from build123d import *

# Parameters (mm, degrees)
ESBO_O1_R                  = 1.35
RESSALTO_EXTRUS_O1_DEPTH   = 2
ESBO_O3_W                  = 40.2
ESBO_O3_H                  = 2
RESSALTO_EXTRUS_O2_DEPTH   = 10.08
ESBO_O4_W                  = 3.1
ESBO_O4_H                  = 12.84
RESSALTO_EXTRUS_O3_DEPTH   = 34
CORTE_EXTRUS_O1_DEPTH      = 55.735280213
CORTE_EXTRUS_O1_DEPTH_BACK = 55.735280213
ESBO_O5_R                  = 1.35
ESBO_O7_W                  = 37.1
ESBO_O7_H                  = 3.24
CORTE_EXTRUS_O2_DEPTH      = 2
RESSALTO_EXTRUS_O5_START   = 2
ESBO_O12_R                 = 1.35
RESSALTO_EXTRUS_O5_DEPTH   = 2
ESBO_O18_W                 = 3.1
ESBO_O18_H                 = 3.24
RESSALTO_EXTRUS_O6_DEPTH   = 2
ESBO_O19_W                 = 3.1
ESBO_O19_H                 = 3.24
RESSALTO_EXTRUS_O7_DEPTH   = 2
ESBO_O21_R                 = 1.301764144
ESBO_O21_R_2               = 1.35
RESSALTO_EXTRUS_O8_DEPTH   = 1.1
RESSALTO_EXTRUS_O9_START   = 1.1
ESBO_O22_R                 = 1.35
RESSALTO_EXTRUS_O9_DEPTH   = 1.1
ESBO_O23_W                 = 3.1
ESBO_O23_H                 = 5.6
RESSALTO_EXTRUS_O10_DEPTH  = 5.85
CORTE_EXTRUS_O3_REACH      = 63.173
ESBO_O24_R                 = 1.35
ESBO_O25_W                 = 4.5
ESBO_O25_H                 = 3.1
CORTE_EXTRUS_O6_DEPTH      = 4.48
ESBO_O27_W                 = 3.1
ESBO_O27_H                 = 29
CORTE_EXTRUS_O7_DEPTH      = 4.48
ESBO_O28_W                 = 25
ESBO_O28_H                 = 40.2
CORTE_EXTRUS_O8_DEPTH      = 1.24
ESBO_O29_W                 = 25
ESBO_O29_H                 = 5.6
RESSALTO_EXTRUS_O11_DEPTH  = 34
ESBO_O31_W                 = 3.1
ESBO_O31_H                 = 25
RESSALTO_EXTRUS_O12_DEPTH  = 2.84
ESBO_O32_W                 = 25
ESBO_O32_H                 = 5.6
RESSALTO_EXTRUS_O13_DEPTH  = 34
FILETE1_R                  = 2.84
ESBO_O33_W                 = 5.6
ESBO_O33_H                 = 3.1
CORTE_EXTRUS_O9_DEPTH      = 0.55
ESBO_O35_W                 = 3.1
ESBO_O35_H                 = 5.6
CORTE_EXTRUS_O10_DEPTH     = 5.03
FILETE2_R                  = 2.8
DIVIDIR1_SURFACE_1_BACK    = 61.888
DIVIDIR1_SURFACE_1_DEPTH   = 123.776
DIVIDIR1_SURFACE_2_BACK    = 61.888
DIVIDIR1_SURFACE_2_DEPTH   = 123.776


with BuildPart() as part:
    # Esboço1 → Ressalto-extrusão1 (new body)
    with BuildSketch(Plane.XY):
        Polygon((0, 0), (5.6, 0), (5.6, -5.85), (34.6, -5.85), (34.6, 0), (40.2, 0), (40.2, -11.45), (0, -11.45), align=None)
        with Locations((2.8, -3.35)):
            Circle(ESBO_O1_R, mode=Mode.SUBTRACT)
        with Locations((37.4, -3.35)):
            Circle(ESBO_O1_R, mode=Mode.SUBTRACT)
        with Locations((31.1, -8.65)):
            Circle(ESBO_O1_R, mode=Mode.SUBTRACT)
        with Locations((9.1, -8.65)):
            Circle(ESBO_O1_R, mode=Mode.SUBTRACT)
    extrude(amount=RESSALTO_EXTRUS_O1_DEPTH)

    # Esboço3 → Ressalto-extrusão2 (add)
    with BuildSketch(Plane.XZ.offset(11.45)):
        with Locations((20.1, 1)):
            Rectangle(ESBO_O3_W, ESBO_O3_H)
    extrude(amount=RESSALTO_EXTRUS_O2_DEPTH)

    # Esboço4 → Ressalto-extrusão3 (add)
    with BuildSketch(Plane(origin=(0, 0, 0), x_dir=(-1, 0, 0), z_dir=(0, 0, -1))):
        with Locations((-38.65, -15.11)):
            Rectangle(ESBO_O4_W, ESBO_O4_H)
        with Locations((-1.55, -15.11)):
            Rectangle(ESBO_O4_W, ESBO_O4_H)
    extrude(amount=RESSALTO_EXTRUS_O3_DEPTH)

    # Esboço5 → Corte-extrusão1 (cut, two sides: drawn at the far end of the back side and taken through both)
    with BuildSketch(Plane.ZY.offset(-37.1).offset(-CORTE_EXTRUS_O1_DEPTH_BACK)):
        with Locations((-6, -14.25)):
            Circle(ESBO_O5_R)
        with Locations((-28, -14.25)):
            Circle(ESBO_O5_R)
    extrude(amount=CORTE_EXTRUS_O1_DEPTH + CORTE_EXTRUS_O1_DEPTH_BACK, mode=Mode.SUBTRACT)

    # Esboço7 → Corte-extrusão2 (cut)
    with BuildSketch(Plane(origin=(0, 0, 0), x_dir=(-1, 0, 0), z_dir=(0, 0, -1))):
        with Locations((-18.55, -19.91)):
            Rectangle(ESBO_O7_W, ESBO_O7_H)
    extrude(amount=-CORTE_EXTRUS_O2_DEPTH, mode=Mode.SUBTRACT)

    # Esboço12 → Ressalto-extrusão5 (add)
    with BuildSketch(Plane(origin=(0, 0, -34), x_dir=(-1, 0, 0), z_dir=(0, 0, -1)).offset(RESSALTO_EXTRUS_O5_START)):
        Polygon((-5.6, 0), (0, 0), (0, -18.29), (-40.2, -18.29), (-40.2, 0), (-34.6, 0), (-34.6, -5.85), (-5.6, -5.85), align=None)
        with Locations(Location((-31.1, -8.65, 0), (0, 0, 180))):
            Circle(ESBO_O12_R, mode=Mode.SUBTRACT)
        with Locations(Location((-9.1, -8.65, 0), (0, 0, 180))):
            Circle(ESBO_O12_R, mode=Mode.SUBTRACT)
        with Locations(Location((-2.8, -3.35, 0), (0, 0, 180))):
            Circle(ESBO_O12_R, mode=Mode.SUBTRACT)
        with Locations(Location((-37.4, -3.35, 0), (0, 0, 180))):
            Circle(ESBO_O12_R, mode=Mode.SUBTRACT)
    extrude(amount=-RESSALTO_EXTRUS_O5_DEPTH)

    # Esboço18 → Ressalto-extrusão6 (add)
    with BuildSketch(Plane.XY):
        with Locations((1.55, -19.91)):
            Rectangle(ESBO_O18_W, ESBO_O18_H)
    extrude(amount=RESSALTO_EXTRUS_O6_DEPTH)

    # Esboço19 → Ressalto-extrusão7 (add)
    with BuildSketch(Plane(origin=(0, 0, -34), x_dir=(-1, 0, 0), z_dir=(0, 0, -1))):
        with Locations((-1.55, -19.91)):
            Rectangle(ESBO_O19_W, ESBO_O19_H)
        with Locations((-38.65, -19.91)):
            Rectangle(ESBO_O19_W, ESBO_O19_H)
    extrude(amount=RESSALTO_EXTRUS_O7_DEPTH)

    # Esboço21 → Ressalto-extrusão8 (add)
    with BuildSketch(Plane.XY.offset(2)):
        Polygon((37.1, -21.53), (40.2, -21.53), (40.2, 0), (34.6, 0), (34.6, -5.85), (5.6, -5.85), (5.6, 0), (0, 0), (0, -21.53), (3.1, -21.53), (3.1, -18.29), (37.1, -18.29), align=None)
        with Locations((2.8, -3.35)):
            Circle(ESBO_O21_R, mode=Mode.SUBTRACT)
        with Locations((9.1, -8.65)):
            Circle(ESBO_O21_R_2, mode=Mode.SUBTRACT)
        with Locations((31.1, -8.65)):
            Circle(ESBO_O21_R_2, mode=Mode.SUBTRACT)
        with Locations((37.4, -3.35)):
            Circle(ESBO_O21_R_2, mode=Mode.SUBTRACT)
    extrude(amount=RESSALTO_EXTRUS_O8_DEPTH)

    # Esboço22 → Ressalto-extrusão9 (add)
    with BuildSketch(Plane(origin=(0, 0, -36), x_dir=(-1, 0, 0), z_dir=(0, 0, -1)).offset(RESSALTO_EXTRUS_O9_START)):
        Polygon((-5.6, 0), (0, 0), (0, -21.53), (-3.1, -21.53), (-3.1, -18.29), (-37.1, -18.29), (-37.1, -21.53), (-40.2, -21.53), (-40.2, 0), (-34.6, 0), (-34.6, -5.85), (-5.6, -5.85), align=None)
        with Locations(Location((-37.4, -3.35, 0), (0, 0, 180))):
            Circle(ESBO_O22_R, mode=Mode.SUBTRACT)
        with Locations(Location((-31.1, -8.65, 0), (0, 0, 180))):
            Circle(ESBO_O22_R, mode=Mode.SUBTRACT)
        with Locations(Location((-9.1, -8.65, 0), (0, 0, 180))):
            Circle(ESBO_O22_R, mode=Mode.SUBTRACT)
        with Locations(Location((-2.8, -3.35, 0), (0, 0, 180))):
            Circle(ESBO_O22_R, mode=Mode.SUBTRACT)
    extrude(amount=-RESSALTO_EXTRUS_O9_DEPTH)

    # Esboço23 → Ressalto-extrusão10 (add)
    with BuildSketch(Plane.XZ.offset(21.53)):
        with Locations((1.55, 0.3)):
            Rectangle(ESBO_O23_W, ESBO_O23_H)
        with Locations((1.55, -34.3)):
            Rectangle(ESBO_O23_W, ESBO_O23_H)
        with Locations((38.65, -34.3)):
            Rectangle(ESBO_O23_W, ESBO_O23_H)
        with Locations((38.65, 0.3)):
            Rectangle(ESBO_O23_W, ESBO_O23_H)
    extrude(amount=RESSALTO_EXTRUS_O10_DEPTH)

    # Corte-extrusão3: up to this face of the body (flat: up to its plane)
    corte_extrus_o3_end = Plane(part.part.faces().sort_by_distance((40.2, -15.177512698, -17))[0])
    # Esboço24 → Corte-extrusão3 (cut, up to the picked face)
    with BuildSketch(Plane.ZY, mode=Mode.PRIVATE) as corte_extrus_o3_sk1:
        with Locations(Location((-34.3, -19.55, 0), (0, 0, 270))):
            Circle(ESBO_O24_R)
    corte_extrus_o3_tool1 = split(extrude(corte_extrus_o3_sk1.sketch, amount=-CORTE_EXTRUS_O3_REACH, mode=Mode.PRIVATE), bisect_by=corte_extrus_o3_end, keep=Keep.BOTH, mode=Mode.PRIVATE)
    # Esboço24 → Corte-extrusão3 (cut, up to the picked face)
    with BuildSketch(Plane.ZY, mode=Mode.PRIVATE) as corte_extrus_o3_sk2:
        with Locations(Location((0.3, -19.55, 0), (0, 0, 270))):
            Circle(ESBO_O24_R)
    corte_extrus_o3_tool2 = split(extrude(corte_extrus_o3_sk2.sketch, amount=-CORTE_EXTRUS_O3_REACH, mode=Mode.PRIVATE), bisect_by=corte_extrus_o3_end, keep=Keep.BOTH, mode=Mode.PRIVATE)
    add(corte_extrus_o3_tool1.solids().sort_by(Axis((0, -19.55, -34.3), (1, 0, 0)))[0], mode=Mode.SUBTRACT)
    add(corte_extrus_o3_tool2.solids().sort_by(Axis((0, -19.55, 0.3), (1, 0, 0)))[0], mode=Mode.SUBTRACT)

    # Esboço25 → Corte-extrusão6 (cut)
    with BuildSketch(Plane.XZ.offset(18.29)):
        with Locations((5.35, -35.55)):
            Rectangle(ESBO_O25_W, ESBO_O25_H)
        with Locations((34.85, -35.55)):
            Rectangle(ESBO_O25_W, ESBO_O25_H)
        with Locations((34.85, 1.55)):
            Rectangle(ESBO_O25_W, ESBO_O25_H)
        with Locations((5.35, 1.55)):
            Rectangle(ESBO_O25_W, ESBO_O25_H)
    extrude(amount=-CORTE_EXTRUS_O6_DEPTH, mode=Mode.SUBTRACT)

    # Esboço27 → Corte-extrusão7 (cut)
    with BuildSketch(Plane.XZ.offset(21.53)):
        with Locations((1.55, -17)):
            Rectangle(ESBO_O27_W, ESBO_O27_H)
        with Locations((38.65, -17)):
            Rectangle(ESBO_O27_W, ESBO_O27_H)
    extrude(amount=-CORTE_EXTRUS_O7_DEPTH, mode=Mode.SUBTRACT)

    # Esboço28 → Corte-extrusão8 (cut)
    with BuildSketch(Plane.XZ.offset(18.29)):
        with Locations((20.1, -17)):
            Rectangle(ESBO_O28_W, ESBO_O28_H)
    extrude(amount=-CORTE_EXTRUS_O8_DEPTH, mode=Mode.SUBTRACT)

    # Esboço29 → Ressalto-extrusão11 (add)
    with BuildSketch(Plane.XY.offset(-34)):
        with Locations((20.1, -14.25)):
            Rectangle(ESBO_O29_W, ESBO_O29_H)
    extrude(amount=RESSALTO_EXTRUS_O11_DEPTH)

    # Esboço31 → Ressalto-extrusão12 (add)
    with BuildSketch(Plane(origin=(0, -8.69, 0), x_dir=(1, 0, 0), z_dir=(0, 1, 0))):
        with Locations((1.55, 17)):
            Rectangle(ESBO_O31_W, ESBO_O31_H)
        with Locations((38.65, 17)):
            Rectangle(ESBO_O31_W, ESBO_O31_H)
    extrude(amount=RESSALTO_EXTRUS_O12_DEPTH)

    # Esboço32 → Ressalto-extrusão13 (add)
    with BuildSketch(Plane.ZY.offset(-37.1)):
        with Locations((-17, -8.65)):
            Rectangle(ESBO_O32_W, ESBO_O32_H)
    extrude(amount=RESSALTO_EXTRUS_O13_DEPTH)

    # Filete1
    filete1_edges = [part.edges().sort_by_distance(p)[0] for p in [
        (32.6, -17.05, -17),
        (7.6, -17.05, -17),
        (20.1, -5.85, -29.5),
        (20.1, -5.85, -4.5),
    ]]
    fillet(filete1_edges, radius=FILETE1_R)

    # Esboço33 → Corte-extrusão9 (cut)
    with BuildSketch(Plane(origin=(0, 0, 0), x_dir=(1, 0, 0), z_dir=(0, 1, 0))):
        with Locations((2.8, 35.55)):
            Rectangle(ESBO_O33_W, ESBO_O33_H)
        with Locations((37.4, 35.55)):
            Rectangle(ESBO_O33_W, ESBO_O33_H)
        with Locations((37.4, -1.55)):
            Rectangle(ESBO_O33_W, ESBO_O33_H)
        with Locations((2.8, -1.55)):
            Rectangle(ESBO_O33_W, ESBO_O33_H)
    extrude(amount=-CORTE_EXTRUS_O9_DEPTH, mode=Mode.SUBTRACT)

    # Esboço35 → Corte-extrusão10 (cut)
    with BuildSketch(Plane.XZ.offset(27.38)):
        with Locations((1.55, 0.3)):
            Rectangle(ESBO_O35_W, ESBO_O35_H)
        with Locations((38.65, 0.3)):
            Rectangle(ESBO_O35_W, ESBO_O35_H)
        with Locations((38.65, -34.3)):
            Rectangle(ESBO_O35_W, ESBO_O35_H)
        with Locations((1.55, -34.3)):
            Rectangle(ESBO_O35_W, ESBO_O35_H)
    extrude(amount=-CORTE_EXTRUS_O10_DEPTH, mode=Mode.SUBTRACT)

    # Filete2
    filete2_edges = [part.edges().sort_by_distance(p)[0] for p in [
        (34.6, -0.55, 1.55),
        (40.2, -0.55, 1.55),
        (0, -0.55, 1.55),
        (5.6, -0.55, 1.55),
        (40.2, -0.55, -35.55),
        (34.6, -0.55, -35.55),
        (5.6, -0.55, -35.55),
        (0, -0.55, -35.55),
        (1.55, -22.35, -31.5),
        (1.55, -22.35, -37.1),
        (38.65, -22.35, -31.5),
        (38.65, -22.35, -37.1),
        (38.65, -22.35, 3.1),
        (38.65, -22.35, -2.5),
        (1.55, -22.35, -2.5),
        (1.55, -22.35, 3.1),
    ]]
    fillet(filete2_edges, radius=FILETE2_R - 0.0001)  # a hair under: the kernel refuses the full size


with BuildPart() as body_2:
    # Dividir1: the piece behind the surface
    add(part.part)
    # Dividir1 surface: a surface, the sketch's curves swept straight by 123.776 mm
    with BuildLine(Plane.XY.offset(3.1).offset(-DIVIDIR1_SURFACE_1_BACK), mode=Mode.PRIVATE) as dividir1_surface_1_path:
        Line((20.1, -0.55), (20.1, -10.85))
        Line((20.1, -10.85), (17.6, -9.85))
        Line((17.6, -9.85), (17.6, -14.85))
        Line((17.6, -14.85), (20.1, -13.85))
        Line((20.1, -13.85), (20.1, -22.35))
    dividir1_surface_1 = Shell.extrude(dividir1_surface_1_path.wire(), (0 * DIVIDIR1_SURFACE_1_DEPTH, 0 * DIVIDIR1_SURFACE_1_DEPTH, 1 * DIVIDIR1_SURFACE_1_DEPTH))
    split(bisect_by=dividir1_surface_1, keep=Keep.BOTTOM)


with BuildPart() as part_1:
    add(part.part)

    # Dividir1: split by a surface, the side it looks to stays
    # Dividir1 surface: a surface, the sketch's curves swept straight by 123.776 mm
    with BuildLine(Plane.XY.offset(3.1).offset(-DIVIDIR1_SURFACE_2_BACK), mode=Mode.PRIVATE) as dividir1_surface_2_path:
        Line((20.1, -0.55), (20.1, -10.85))
        Line((20.1, -10.85), (17.6, -9.85))
        Line((17.6, -9.85), (17.6, -14.85))
        Line((17.6, -14.85), (20.1, -13.85))
        Line((20.1, -13.85), (20.1, -22.35))
    dividir1_surface_2 = Shell.extrude(dividir1_surface_2_path.wire(), (0 * DIVIDIR1_SURFACE_2_DEPTH, 0 * DIVIDIR1_SURFACE_2_DEPTH, 1 * DIVIDIR1_SURFACE_2_DEPTH))
    split(bisect_by=dividir1_surface_2, keep=Keep.TOP)


solid = body_2.part
Work out the finished part from the listing and answer in its coordinate system (mm). A direction names the side the tool comes from. Coordinates: 2 decimals unless noted, no trailing zeros. Write each loop counter-clockwise with the first axis right and the second up, starting at its lowest first coordinate (ties: lowest second). Pieces come first, ordered by that corner, then holes. Notation, with made-up numbers: M 73,38.25 L 80,38.25 A9 ccw 80,42.25 Z; hole C 54.5,48 d10. An arc over 180 degrees is marked long. Use one line per item in the form item = value. Start each with the question number.
1. The part is cut by section B-B (y = -6.25). Give the vertices of the cut face in (x, z), plus the area to 3 significant figures.
2. The mould has two halves that part along Z. Classify faces 1 (the face through (10.191, -6.704, -28.69)), 2 (the face through (18.87, -10.36, -35.57)): released by +Z, released by -Z, zero draft, split by the parting line, or undercut.
3. Each of these flat-tipped pins is pushed along its axis until it touches: P1, Ø2, axis at x = 5, y = -16, coming from the -Z side; P2, Ø0.8, axis at y = -4.5, z = 2, coming from the +X side; P3, Ø5, axis at x = 17, z = -2.5, coming from the -Y side; P4, Ø3.5, axis at x = 15, z = 1, coming from the +Y side. Where does it stop, or does it pass through?
4. The part is cut by section A-A (x = 18.75). Give the vertices of the cut face in (y, z).
5. The part is cut by section C-C (z = -13). Give the vertices of the cut face in (x, y).
6. The part is cut by section D-D (x = 9.1). Give the vertices of the cut face in (y, z).
7. A tool of negligible diameter and unlimited length cuts with its end or side. For faces 3 (the face through (1.45, -3.41, -35.57)), 4 (the face through (8.41, -16.196, -16.719)), 5 (the face through (13, -11.45, -2)), from which of +Z, -Z, +X, -X, +Y, -Y can it reach the whole face along a straight path? Write none if from no direction.
8. Straight lines are drawn through the part: probe 1 along Z at (x, y) = (15.5, -10.25); probe 2 along Z at (x, y) = (1.8, -14.25); probe 3 along Z at (x, y) = (2.75, -19). For each, find the intervals that lie inside material, in ascending order. Write a range as from..to.
Evaluation:
q1.outline = M 0,-37.1 L 20.1,-37.1 L 20.1,-34 L 0,-34 Z; M 0,-28.11 L 20.1,-28.11 L 20.1,-5.89 L 0,-5.89 Z; M 0,0 L 20.1,0 L 20.1,3.1 L 0,3.1 Z
q1.area = 571 mm^2
q2.face_1 = undercut
q2.face_2 = zero draft
q3.P1 = through
q3.P2 = 5.6
q3.P3 = -17.05
q3.P4 = -5.85
q4.outline = M -17.05,-37.1 L -14.39,-37.1 L -14.39,3.1 L -17.05,3.1 Z; M -10.31,-37.1 L -5.85,-37.1 L -5.85,-34 L -10.31,-34 Z; M -10.31,-29.5 L -8.69,-29.5 A2.84 ccw -5.85,-26.66 L -5.85,-7.34 A2.84 ccw -8.69,-4.5 L -10.31,-4.5 Z; M -10.31,0 L -5.85,0 L -5.85,3.1 L -10.31,3.1 Z
q5.outline = M 0,-17.05 L 3.1,-17.05 L 3.1,-11.45 L 7.6,-11.45 L 7.6,-14.21 A2.84 ccw 10.44,-17.05 L 20.1,-17.05 L 20.1,-13.85 L 17.6,-14.85 L 17.6,-9.85 L 20.1,-10.85 L 20.1,-5.85 L 0,-5.85 Z
q6.outline = M -16.71,-37.1 L -10,-37.1 L -10,-34 L -11.45,-34 L -11.45,-29.5 L -8.69,-29.5 A2.84 ccw -5.85,-26.66 L -5.85,-7.34 A2.84 ccw -8.69,-4.5 L -11.45,-4.5 L -11.45,0 L -10,0 L -10,3.1 L -16.71,3.1 Z; M -7.3,-37.1 L -5.85,-37.1 L -5.85,-34 L -7.3,-34 Z; M -7.3,0 L -5.85,0 L -5.85,3.1 L -7.3,3.1 Z
q7.face_3 = -Z
q7.face_4 = +Z, -Z, -Y
q7.face_5 = +X, +Y
q8.probe_1 = -37.1..-34, -29.5..-4.5, 0..3.1
q8.probe_2 = -37.1..-29.35, -26.65..-7.35, -4.65..3.1
q8.probe_3 = -37.1..-35.53, -33.07..-31.5, -2.5..-0.93, 1.53..3.1
